Could you check a few things on this model? Use its own coordinates, in mm. A direction names the side the tool comes from. Coordinates: 2 decimals unless noted, no trailing zeros. Write each loop counter-clockwise with the first axis right and the second up, starting at its lowest first coordinate (ties: lowest second). Pieces come first, ordered by that corner, then holes. Notation, with made-up numbers: M -27,-35 L 18,-35 A6 ccw 18,-31 Z; hole C -2.75,81.25 d7. An arc over 180 degrees is marked long. Write item = value, one per line.
```python
from build123d import *

# Parameters (mm, degrees)
SKETCH1_R           = 20
SKETCH1_R_2         = 10
BOSS_EXTRUDE2_DEPTH = 20
BOSS_EXTRUDE3_START = 10
SKETCH2_R           = 20
SKETCH2_R_2         = 10
BOSS_EXTRUDE3_DEPTH = 10
SKETCH3_W           = 15
SKETCH3_H           = 5
BOSS_EXTRUDE4_DEPTH = 120


with BuildPart() as part:
    # Sketch1 → Boss-Extrude2 (new body)
    # profile 1 of 2: a face of its own
    with BuildSketch(Plane(origin=(0, 0, 0), x_dir=(0, 0, -1), z_dir=(1, 0, 0))):
        with BuildLine():
            Line((-55.154478161, 25), (-55.154478161, 0))
            Line((-55.154478161, 0), (64.845521839, 0))
            Line((64.845521839, 0), (64.845521839, 25))
            Line((64.845521839, 25), (49.845521839, 25))
            Line((49.845521839, 25), (21.950490606, 45.270819657))
            ThreePointArc((21.950490606, 45.270819657), (24.06645602, 40.32794394), (24.789189269, 35))
            ThreePointArc((24.789189269, 35), (-0.58635613, 15.735952874), (-12.321161896, 45.35547599))
            Line((-12.321161896, 45.35547599), (-40.154478161, 25))
            Line((-40.154478161, 25), (-55.154478161, 25))
        make_face()
    # profile 2 of 2: a face of its own
    with BuildSketch(Plane(origin=(0, 0, 0), x_dir=(0, 0, -1), z_dir=(1, 0, 0))):
        with Locations((4.789189269, 35)):
            Circle(SKETCH1_R)
        with Locations((4.789189269, 35)):
            Circle(SKETCH1_R_2, mode=Mode.SUBTRACT)
    extrude(amount=-BOSS_EXTRUDE2_DEPTH)

    # Sketch2 → Boss-Extrude3 (add)
    with BuildSketch(Plane(origin=(0, 0, 0), x_dir=(0, 0, -1), z_dir=(1, 0, 0)).offset(BOSS_EXTRUDE3_START)):
        with Locations((4.789189269, 35)):
            Circle(SKETCH2_R)
        with Locations((4.789189269, 35)):
            Circle(SKETCH2_R_2, mode=Mode.SUBTRACT)
    extrude(amount=-BOSS_EXTRUDE3_DEPTH)

    # Sketch3 → Boss-Extrude4 (add)
    with BuildSketch(Plane.XY.offset(55.154478161)):
        with Locations((-27.5, 2.5)):
            Rectangle(SKETCH3_W, SKETCH3_H)
    extrude(amount=-BOSS_EXTRUDE4_DEPTH)

    # Mirror1: part across plane


with BuildPart() as part_1:
    add(part.part)
    add(part.part.mirror(Plane.ZY.offset(35)))


solid = part_1.part
```
Item 1: Imagine slicing it at D-D (y = 41.5). Write out the boundary of the cut face in (x, z).
Numbers:
outline = M -80,-23.7 L -70,-23.7 L -70,-27.14 L -50,-27.14 L -50,-12.39 L -80,-12.39 Z; M -80,2.81 L -50,2.81 L -50,17.59 L -70,17.59 L -70,14.13 L -80,14.13 Z; M -20,-27.14 L 0,-27.14 L 0,-23.7 L 10,-23.7 L 10,-12.39 L -20,-12.39 Z; M -20,2.81 L 10,2.81 L 10,14.13 L 0,14.13 L 0,17.59 L -20,17.59 Z
Item 2: Imagine slicing it at B-B (y = 13). Write out the boundary of the cut face in (x, z).
Numbers:
outline = M -70,-64.85 L -50,-64.85 L -50,55.15 L -70,55.15 Z; M -20,-64.85 L 0,-64.85 L 0,55.15 L -20,55.15 Z
Item 3: If I drill on line 1 along X through (y, z) = (48, -14); line 2 along X through (y, z) = (15.5, 50); line 3 along X through (y, z) = (3.5, -50), over which ranges is the centre line in solid material (lowest first)?
Numbers:
line_1 = -80 to -50, -20 to 10
line_2 = -70 to -50, -20 to 0
line_3 = -70 to 0
Item 4: Imagine slicing it at C-C (z = 3). Write out the boundary of the cut face in (x, y), and give its area (3 significant figures).
Numbers:
outline = M -80,16.58 L -70,16.58 L -70,0 L 0,0 L 0,16.58 L 10,16.58 L 10,28.73 L -20,28.73 L -20,5 L -50,5 L -50,28.73 L -80,28.73 Z; M -80,41.27 L -50,41.27 L -50,53.42 L -80,53.42 Z; M -20,41.27 L 10,41.27 L 10,53.42 L -20,53.42 Z
area = 2,270 mm²
Item 5: For faces 5 (the face through (-60, 25, -57)), 6 (the face through (-35, 5, -4)), 7 (the face through (-60, 25, 48)), which set-ups out of +Z, -Z, +X, -X, +Y, -Y let a thin tool reach every point of the face, with its end or its side?
Numbers:
face_5 = -Z, +X, -X, +Y
face_6 = +Z, -Z, +Y
face_7 = +Z, +X, -X, +Y
Item 6: I'm going to push flat-ended pins straight in: P1, Ø4, axis at x = 0.5, z = 26.5, coming from the +Y side; P2, Ø4, axis at y = 16, z = -17.5, coming from the +X side; P3, Ø9, axis at x = -33.5, z = -20, coming from the +Y side. Where does each tip first touch, or does it pass through?
Numbers:
P1 = 36.4
P2 = 0
P3 = 5
Item 7: Imagine slicing it at A-A (x = -58). Write out the boundary of the cut face in (y, z).
Numbers:
outline = M 0,-64.85 L 25,-64.85 L 25,-49.85 L 45.27,-21.95 A20 ccw 45.36,12.32 L 25,40.15 L 25,55.15 L 0,55.15 Z; hole C 35,-4.79 d20
Item 8: If we mould it in two halves opening along Y, with no side actions, what happens to faces 1 (the face through (-10, 25, 48)), 2 (the face through (-68.54, 54.83, -2.19)), 3 (the face through (-4.79, 25.24, -2.62)), 4 (the face through (0, 13, -4))? For each: pulls with the +Y half, pulls with the -Y half, needs draft (parallel to the pull), parting line crosses it, or undercut.
Numbers:
face_1 = pulls with the +Y half
face_2 = parting line crosses it
face_3 = undercut
face_4 = needs draft
